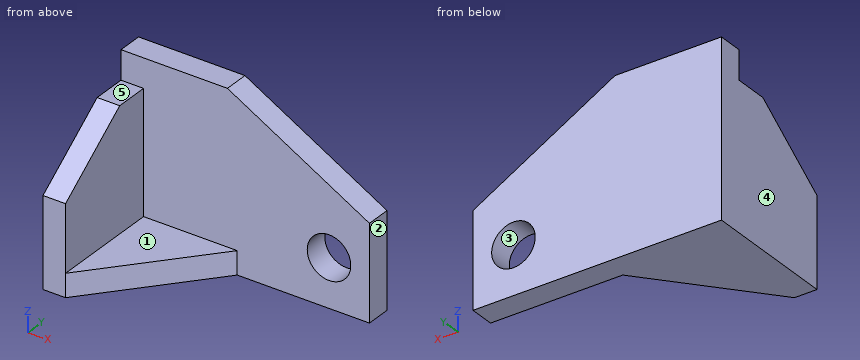
from build123d import *

# Parameters (mm, degrees)
F0_W      = 108.6182296276
F0_H      = 59.0771511197
F1_DEPTH  = 25.4
F2_W      = 108.6182296276
F2_H      = 10.8553785831
F3_DEPTH  = 50.8
F4_W      = 9.8601616919
F4_H      = 48.2217725366
F5_DEPTH  = 38.1
F7_DEPTH  = 25.4
F9_DEPTH  = 25.4
F11_DEPTH = 25.4
F13_D     = 19.05
F14_DEPTH = 15.24
F16_DEPTH = 15.24


with BuildPart() as f1:
    # F0 (on Top) → F1 (new body)
    with BuildSketch(Plane.XY):
        with Locations((3.4888088703, -3.9539821446)):
            Rectangle(F0_W, F0_H)
    extrude(amount=F1_DEPTH)

    # F2 (on face) → F3 (join)
    with BuildSketch(Plane.XY.offset(25.4)):
        with Locations((3.4888088703, 20.1569041237)):
            Rectangle(F2_W, F2_H)
    extrude(amount=F3_DEPTH)

    # F4 (on face) → F5 (join)
    with BuildSketch(Plane.XY.offset(25.4)):
        with Locations((-45.8902250975, -9.3816714361)):
            Rectangle(F4_W, F4_H)
    extrude(amount=F5_DEPTH)

    # F6 (on face) → F7 (cut)
    with BuildSketch(Plane.YZ.offset(-40.9601442516)):
        Polygon((-33.4925577044, 39.1064621508), (0, 63.5), (-33.4925577044, 63.5), align=None)
    extrude(amount=-F7_DEPTH, mode=Mode.SUBTRACT)

    # F8 (on face) → F9 (cut)
    with BuildSketch(Plane.XY.offset(25.4)):
        Polygon((57.7979236841, 14.7292148322), (0, 14.7292148322), (-40.9601442516, -33.4925577044), (57.7979236841, -33.4925577044), align=None)
    extrude(amount=-F9_DEPTH, mode=Mode.SUBTRACT)

    # F10 (on face) → F11 (cut)
    with BuildSketch(Plane.XZ.offset(-14.7292148322)):
        Polygon((57.7979236841, 76.2), (-4.3028630316, 76.2), (57.7979236841, 41.5174737573), align=None)
    extrude(amount=-F11_DEPTH, mode=Mode.SUBTRACT)

    # F13 (through all)
    with Locations(Plane.XZ.offset(-14.7292148322)):
        with Locations((40.121294558, 21.1239363998)):
            Hole(F13_D / 2)

    # F14 (add): a face of the model
    f14_faces = [f1.faces().sort_by_distance(p)[0] for p in [
        (-27.3067628344, -1.3447093467, 25.4),
    ]]
    extrude(f14_faces, amount=-F14_DEPTH)

    # F15 (on face) → F16 (cut)
    with BuildSketch(Plane.XY.offset(25.4)):
        Polygon((0, 14.7292148322), (-40.9601442516, 14.7292148322), (-40.9601442516, -33.4925577044), align=None)
    extrude(amount=-F16_DEPTH, mode=Mode.SUBTRACT)


solid = f1.part
The listing builds one solid part. Answer for the finished solid, in the listing's coordinates (mm). Face numbers are marked on the shaded views. A direction names the side the tool comes from. Coordinates: 2 decimals unless noted, no trailing zeros. Order: outer loops, then holes, each group sorted by start corner. A loop starts at its lowest first (then second) coordinate and runs counter-clockwise, first axis right, second up.
Q1. For a pull along Z with two mould halves and no side action, classify the marked faces 3, 4 and 5 as pulls with the +Z half, pulls with the -Z half, needs draft (parallel to the pull), parting line crosses it, or undercut.
Q2. Consider line 1 (Y direction, x = -11, z = 69); line 2 (Z direction, x = -18, y = 6.5); line 3 (X direction, y = 8, z = 62). Determine where each line is inside the solid, lowest interval first.
Q3. A cutting plane is placed at D-D, the plane y = 7.5. Write down the section's boundary in (x, z), and give its area (3 significant figures).
Q4. A cutting plane is placed at C-C, the plane y = 17. Write down the section's boundary in (x, z) (3 decimals).
Q5. Which of the six approach directions +Z, -Z, +X, -X, +Y, -Y give full straight-line access (tool end or side, diameter ignored) to the marked faces 1 and 2?
Q6. A cutting plane is placed at A-A, the plane x = -43. Write down the section's boundary in (y, z).
Q7. A cutting plane is placed at B-B, the plane z = 32. Write down the section's boundary in (x, y), and give its area (3 significant figures).
Q8. Given P1, Ø5, axis at y = -3.5, z = 61.5, coming from the +X side; P2, Ø20.5, axis at x = -20, y = -8.5, coming from the +Z side; P3, Ø3, axis at y = 18.5, z = 64.5, coming from the +X side, each flat-ended and moving along its own axis, determine where each tip first touches the part or whether it passes through.
Answers follow:
1. face 3: undercut
1. face 4: needs draft
1. face 5: pulls with the +Z half
2. line 1: y = 14.73 to 25.58
2. line 2: z = 0 to 10.16
2. line 3: x = -50.82 to -40.96
3. outline: (-50.82, 0) - (-6.14, 0) - (-6.14, 10.16) - (-40.96, 10.16) - (-40.96, 63.5) - (-50.82, 63.5) - close
3. area: 980 mm2
4. outline: (-50.82, 0) - (57.798, 0) - (57.798, 41.517) - (-4.303, 76.2) - (-50.82, 76.2) - close; hole circle Ø19.05 at (40.121, 21.124)
5. face 1: +Z, +X, -Y
5. face 2: +Z, -Z, +X, +Y, -Y
6. outline: (-33.49, 0) - (25.58, 0) - (25.58, 76.2) - (14.73, 76.2) - (14.73, 63.5) - (0, 63.5) - (-33.49, 39.11) - close
7. outline: (-50.82, -33.49) - (-40.96, -33.49) - (-40.96, 14.73) - (57.8, 14.73) - (57.8, 25.58) - (-50.82, 25.58) - close
7. area: 1,650 mm2
8. P1: stops at x = -40.96
8. P2: stops at z = 10.16
8. P3: stops at x = 19.33
